Check sheet for the drawn part. Datum: minimum x, y, z corner. Units: mm. A direction names the side the tool comes from. Coordinates: 2 decimals unless noted, no trailing zeros. Write each loop counter-clockwise with the first axis right and the second up, starting at its lowest first coordinate (ties: lowest second). Pieces come first, ordered by that corner, then holes. Notation, with made-up numbers: (29.25, -14.75) - (71.25, -14.75) arc R21 ccw to (71.25, 14.25) - close; hole circle Ø2 at (-23, 15.5). An arc over 180 degrees is marked (long way). Use one line per item in the form item = value. Start each with the question number.
1. Cross-section at A-A on y = 4.5. Record the boundary of the cut face in (x, z), then the cut area to 3 significant figures.
2. Draft check along Z on the marked faces 4, 5 and 6. Enter one of: +Z half, -Z half, draft (parallel to the pull), parting line (faces both ways), or undercut.
3. Cross-section at C-C on z = 7. Record the boundary of the cut face in (x, y), then the cut area to 3 significant figures.
4. Scan lines: line 1 along Z through (x, y) = (9.9, 4.5); line 2 along X through (y, z) = (7.5, 5); line 3 along X through (y, z) = (1.5, 3). Record each from-to range of solid material in increasing order.
5. Go/stop test with flat-tipped pins: pin 1 Ø2.5 at (y, z) = (4.5, 4.5) entering from +X; pin 2 Ø1 at (x, y) = (2, 7.5) entering from -Z; pin 3 Ø5 at (x, y) = (9.5, 8) entering from -Z; pin 4 Ø1 at (x, z) = (3.5, 2) entering from +Y. Record where each tip stops, or that it passes through.
6. Cross-section at B-B on z = 4.5. Record the boundary of the cut face in (x, y).
7. Cross-section at D-D on x = 6.5. Record the boundary of the cut face in (y, z).
8. Tool access check on the marked faces 1, 2 and 3. Record the directions out of +Z, -Z, +X, -X, +Y, -Y that give a thin tool (end or side, any length) a straight path to the whole face; none if there is none.
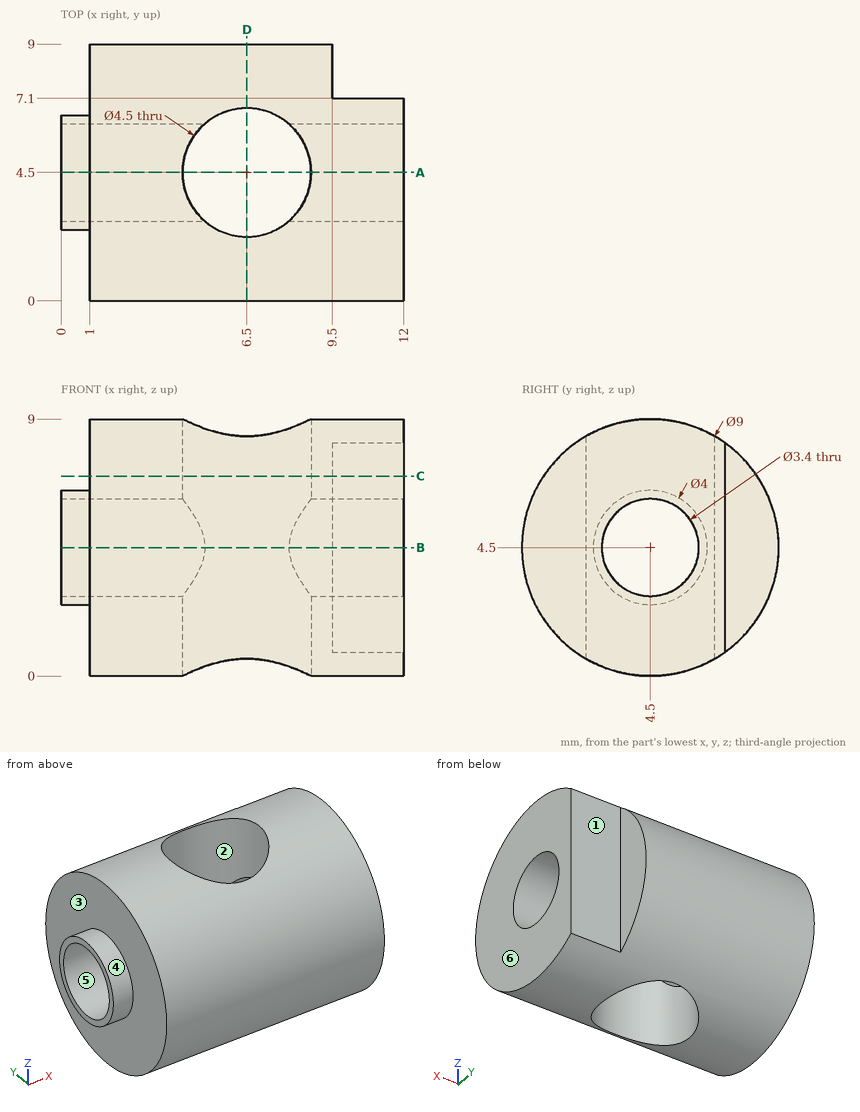
Final values:
q1.outline = (0, 2.5) - (1, 2.5) - (1, 0) - (4.25, 0) - (4.25, 2.8) - (0, 2.8) - close; (0, 6.2) - (4.25, 6.2) - (4.25, 9) - (1, 9) - (1, 6.5) - (0, 6.5) - close; (8.75, 0) - (12, 0) - (12, 2.8) - (8.75, 2.8) - close; (8.75, 6.2) - (12, 6.2) - (12, 9) - (8.75, 9) - close
q1.area = 37.0 mm²
q2.face_4 = parting line
q2.face_5 = undercut
q2.face_6 = draft
q3.outline = (1, 0.76) - (12, 0.76) - (12, 7.1) - (9.5, 7.1) - (9.5, 8.24) - (1, 8.24) - close; hole circle Ø4.5 at (6.5, 4.5)
q3.area = 63.6 mm²
q4.line_1 = 0 to 2.8, 6.2 to 9
q4.line_2 = 1 to 9.5
q4.line_3 = 1 to 12
q5.pin_1 = through
q5.pin_2 = 0.76
q5.pin_3 = 0.11
q5.pin_4 = 8.53
q6.outline = (0, 2.5) - (1, 2.5) - (1, 0) - (12, 0) - (12, 2.8) - (7.97, 2.8) arc R2.25 cw to (5.03, 2.8) - (0, 2.8) - close; (0, 6.2) - (5.03, 6.2) arc R2.25 cw to (7.97, 6.2) - (12, 6.2) - (12, 7.1) - (9.5, 7.1) - (9.5, 9) - (1, 9) - (1, 6.5) - (0, 6.5) - close
q7.outline = (2.25, 0.6) - (2.25, 8.4) arc R4.5 ccw to start; (6.75, 0.6) arc R4.5 ccw to (6.75, 8.4) - close
q8.face_1 = +Z, -Z, +X, +Y
q8.face_2 = +Z, -Z
q8.face_3 = -X
